Drawing for the job (mm, zero at the part's lowest x, y, z). A direction names the side the tool comes from. Coordinates: 2 decimals unless noted, no trailing zeros. Write each loop counter-clockwise with the first axis right and the second up, starting at its lowest first coordinate (ties: lowest second). Pieces come first, ordered by that corner, then holes. Notation, with made-up numbers: (-4.75, 87.25) -> (23.25, 87.25) arc R25 cw to (23.25, 115.25) -> close; hole circle Ø4 at (86.5, 80). An arc over 180 degrees is marked (long way). Answer as CSV lines item,"result".
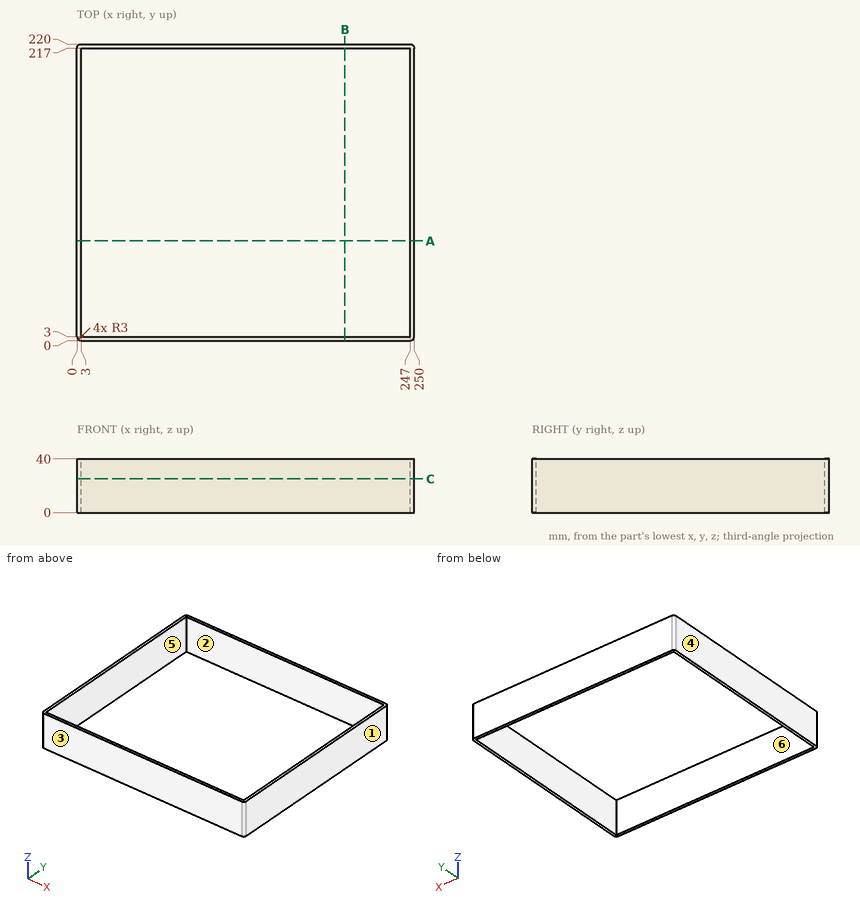
Item 1: 3-axis set-ups, long thin cutter, end or side, ignore diameter. For the marked faces 1 and 2: which of +Z, -Z, +X, -X, +Y, -Y reach the whole face in a straight line?
Answer below:
face 1,"+Z, -Z, +X, +Y, -Y"
face 2,"+Z, -Z"
Item 2: Saw through at B-B on x = 198.5. Give the cut face in (y, z).
Answer below:
outline,"(0, 0) -> (3, 0) -> (3, 40) -> (0, 40) -> close; (217, 0) -> (220, 0) -> (220, 40) -> (217, 40) -> close"
Item 3: Two-plate mould, pull along Y, no slides. Class the marked faces 3, 4, 5 and 6: pulls with the +Y half, pulls with the -Y half, needs draft (parallel to the pull), parting line crosses it, or undercut.
Answer below:
face 3,"pulls with the -Y half"
face 4,"needs draft"
face 5,"undercut"
face 6,"undercut"
Item 4: Wall check: line 1 (Y direction, x = 174, z = 5.5); line 2 (X direction, y = 206.5, z = 3). Give the ranges that are in metal, low to high. Write a range as from..to.
Answer below:
line 1,"y = 0..3, 217..220"
line 2,"x = 0..3, 247..250"
Item 5: Saw through at C-C on z = 25. Give the cut face in (x, y).
Answer below:
outline,"(0, 3) arc R3 ccw to (3, 0) -> (247, 0) arc R3 ccw to (250, 3) -> (250, 217) arc R3 ccw to (247, 220) -> (3, 220) arc R3 ccw to (0, 217) -> close; hole (3, 3) -> (247, 3) -> (247, 217) -> (3, 217) -> close"
Item 6: Saw through at A-A on y = 74. Give the cut face in (x, z), and give its area (3 significant figures).
Answer below:
outline,"(0, 0) -> (3, 0) -> (3, 40) -> (0, 40) -> close; (247, 0) -> (250, 0) -> (250, 40) -> (247, 40) -> close"
area,"240 mm2"
